Can you work these out from the model? Positions are in its coordinate system, mm. Face numbers are marked on the shaded views. A direction names the side the tool comes from. Give positions to 0.01 mm unless a question says otherwise; leave off trailing zeros. Order: outer loops, then holes, each group sorted by start corner. A loop starts at its lowest first (then second) coordinate and runs counter-clockwise, first axis right, second up. Notation, with made-up numbers: (84, 15.25) - (141, 15.25) arc R25 ccw to (141, 54.25) - close; hole circle Ø4 at (-5, 66.5). An arc over 180 degrees is marked (long way). Return JSON: item names as keys, results as strings.
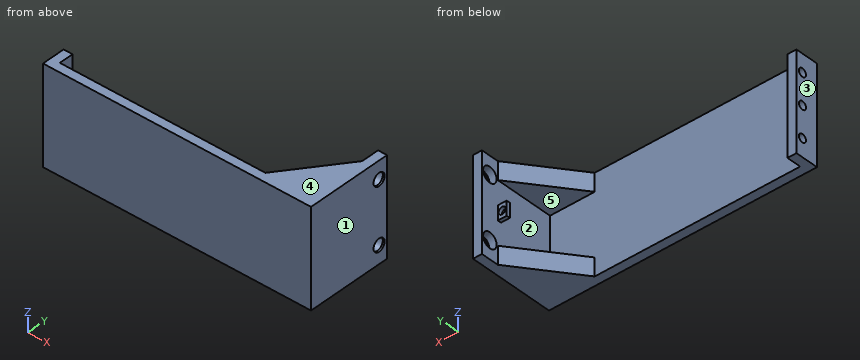
```python
from build123d import *

# Parameters (mm, degrees)
SKETCH1_W                 = 150
SKETCH1_H                 = 54.5
BOSS_EXTRUDE1_DEPTH       = 5
SKETCH2_W                 = 5
SKETCH2_H                 = 54.5
BOSS_EXTRUDE2_DEPTH       = 8
F_8_CLEARANCE_HOLE1_D     = 4.4958
F_8_CLEARANCE_HOLE1_DEPTH = 17
F_8_CLEARANCE_HOLE1_TIP   = 1.350674586
SKETCH7_W                 = 5
SKETCH7_H                 = 54.5
BOSS_EXTRUDE3_DEPTH       = 43
SKETCH8_R                 = 4.25
CUT_EXTRUDE1_DEPTH        = 4
RIB1_REACH                = 120.085
SKETCH10_WALL_W           = 279.571445908
SKETCH10_WALL_H           = 10
RIB3_REACH                = 120.085
SKETCH12_WALL_W           = 279.571445908
SKETCH12_WALL_H           = 10
SKETCH13_W                = 8
SKETCH13_H                = 2
BOSS_EXTRUDE4_DEPTH       = 5
SKETCH14_R                = 2
CUT_EXTRUDE2_DEPTH        = 2
SKETCH15_R                = 3.5
CUT_EXTRUDE3_DEPTH        = 1


with BuildPart() as part:
    # Sketch1 → Boss-Extrude1 (new body)
    with BuildSketch(Plane(origin=(0, 0, 0), x_dir=(1, 0, 0), z_dir=(0, 1, 0))):
        with Locations((-18.112463826, -1.689393939)):
            Rectangle(SKETCH1_W, SKETCH1_H)
    extrude(amount=BOSS_EXTRUDE1_DEPTH)

    # Sketch2 → Boss-Extrude2 (add)
    with BuildSketch(Plane(origin=(0, 5, 0), x_dir=(1, 0, 0), z_dir=(0, 1, 0))):
        with Locations((-90.612463826, -1.689393939)):
            Rectangle(SKETCH2_W, SKETCH2_H)
    extrude(amount=BOSS_EXTRUDE2_DEPTH)

    # #8 Clearance Hole1
    with Locations(Plane(origin=(-93.112463826, 9.2, -15.560606061), x_dir=(0, 0, -1), z_dir=(-1, 0, 0))):
        with Locations((0, 0), (-17.25, 0), (-34.5, 0)):
            Hole(F_8_CLEARANCE_HOLE1_D / 2, depth=F_8_CLEARANCE_HOLE1_DEPTH)
            with Locations((0, 0, -(F_8_CLEARANCE_HOLE1_DEPTH + F_8_CLEARANCE_HOLE1_TIP / 2))):  # 118° drill point
                Cone(0, F_8_CLEARANCE_HOLE1_D / 2, F_8_CLEARANCE_HOLE1_TIP, mode=Mode.SUBTRACT)

    # Sketch7 → Boss-Extrude3 (add)
    with BuildSketch(Plane(origin=(0, 5, 0), x_dir=(1, 0, 0), z_dir=(0, 1, 0))):
        with Locations((54.387536174, -1.689393939)):
            Rectangle(SKETCH7_W, SKETCH7_H)
    extrude(amount=BOSS_EXTRUDE3_DEPTH)

    # Sketch8 → Cut-Extrude1 (cut)
    with BuildSketch(Plane.ZY.offset(-51.887536174)):
        with Locations((-15.560606061, 43)):
            Circle(SKETCH8_R)
        with Locations((18.939393939, 43)):
            Circle(SKETCH8_R)
    extrude(amount=-CUT_EXTRUDE1_DEPTH, mode=Mode.SUBTRACT)

    # Sketch10 wall → Rib1 (add, up to next)
    with BuildSketch(Plane(origin=(39.387536174, 21.5, -25.560606061), x_dir=(-0.603857687995, -0.797092148154, 0), z_dir=(-0.797092148154, 0.603857687995, 0)), mode=Mode.PRIVATE) as rib1_sk1:
        with Locations((0, 5)):
            Rectangle(SKETCH10_WALL_W, SKETCH10_WALL_H)
    rib1_tool1 = extrude(rib1_sk1.sketch, amount=-RIB1_REACH, mode=Mode.PRIVATE) - part.part
    add(rib1_tool1.solids().sort_by_distance((39.387536174, 21.5, -25.560606061))[0])

    # Sketch12 wall → Rib3 (add, up to next)
    with BuildSketch(Plane(origin=(39.387536174, 21.5, 28.939393939), x_dir=(-0.603857687995, -0.797092148154, 0), z_dir=(0.797092148154, -0.603857687995, 0)), mode=Mode.PRIVATE) as rib3_sk1:
        with Locations((0, 5)):
            Rectangle(SKETCH12_WALL_W, SKETCH12_WALL_H)
    rib3_tool1 = extrude(rib3_sk1.sketch, amount=RIB3_REACH, mode=Mode.PRIVATE) - part.part
    add(rib3_tool1.solids().sort_by_distance((39.387536174, 21.5, 28.939393939))[0])

    # Sketch13 → Boss-Extrude4 (add)
    with BuildSketch(Plane.ZY.offset(-51.887536174)):
        with Locations((1.689393939, 37)):
            Rectangle(SKETCH13_W, SKETCH13_H)
    extrude(amount=BOSS_EXTRUDE4_DEPTH)

    # Sketch14 → Cut-Extrude2 (cut)
    with BuildSketch(Plane(origin=(0, 38, 0), x_dir=(1, 0, 0), z_dir=(0, 1, 0))):
        with Locations(Location((49.387536174, -1.689393939, 0), (0, 0, 270))):
            Circle(SKETCH14_R)
    extrude(amount=-CUT_EXTRUDE2_DEPTH, mode=Mode.SUBTRACT)

    # Sketch15 → Cut-Extrude3 (cut)
    with BuildSketch(Plane.ZY.offset(-55.887536174)):
        with Locations((-15.560606061, 43)):
            Circle(SKETCH15_R)
        with Locations((18.939393939, 43)):
            Circle(SKETCH15_R)
    extrude(amount=-CUT_EXTRUDE3_DEPTH, mode=Mode.SUBTRACT)


solid = part.part
```
1. Suppose I cut it at B-B (z = 11.5). List the corners of the cut face in (x, y) for me.
Checks:
{"outline": "(-93.11, 0) - (56.89, 0) - (56.89, 48) - (51.89, 48) - (51.89, 5) - (-88.11, 5) - (-88.11, 13) - (-93.11, 13) - close"}
2. Suppose I cut it at C-C (z = 1.5). List the corners of the cut face in (x, y) for me.
Checks:
{"outline": "(-93.11, 0) - (56.89, 0) - (56.89, 48) - (51.89, 48) - (51.89, 38) - (51.38, 38) - (51.38, 36) - (51.89, 36) - (51.89, 5) - (-88.11, 5) - (-88.11, 6.96) - (-93.11, 6.96) - close; (-93.11, 11.44) - (-88.11, 11.44) - (-88.11, 13) - (-93.11, 13) - close; (46.89, 36) - (47.4, 36) - (47.4, 38) - (46.89, 38) - close"}
3. Suppose I cut it at A-A (y = 43). List the corners of the cut face in (x, z) for me.
Checks:
{"outline": "(51.89, -25.56) - (56.89, -25.56) - (56.89, -19.06) - (55.89, -19.06) - (55.89, -19.81) - (51.89, -19.81) - close; (51.89, -11.31) - (55.89, -11.31) - (55.89, -12.06) - (56.89, -12.06) - (56.89, 15.44) - (55.89, 15.44) - (55.89, 14.69) - (51.89, 14.69) - close; (51.89, 23.19) - (55.89, 23.19) - (55.89, 22.44) - (56.89, 22.44) - (56.89, 28.94) - (51.89, 28.94) - close"}
4. If I drill on L1, parallel to Z at x = -91, y = 9.2; L2, parallel to Z at x = 51, y = 22; L3, parallel to Y at x = 17.5, z = -6, over which ranges is the centre line in solid material (lowest first)? Write a range as [from, to].
Checks:
{"L1": "[-25.56, -17.81], [-13.31, -0.56], [3.94, 16.69], [21.19, 28.94]", "L2": "[-25.56, -15.56], [18.94, 28.94]", "L3": "[0, 5]"}
5. Suppose I cut it at D-D (y = 9.2). List the corners of the cut face in (x, z) for me.
Checks:
{"outline": "(-93.11, -25.56) - (-88.11, -25.56) - (-88.11, -17.81) - (-93.11, -17.81) - close; (-93.11, -13.31) - (-88.11, -13.31) - (-88.11, -0.56) - (-93.11, -0.56) - close; (-93.11, 3.94) - (-88.11, 3.94) - (-88.11, 16.69) - (-93.11, 16.69) - close; (-93.11, 21.19) - (-88.11, 21.19) - (-88.11, 28.94) - (-93.11, 28.94) - close; (30.07, -25.56) - (56.89, -25.56) - (56.89, 28.94) - (30.07, 28.94) - (30.07, 18.94) - (51.89, 18.94) - (51.89, -15.56) - (30.07, -15.56) - close"}
6. On a 3-axis mill with a long thin cutter (end or side, diameter ignored), from which of +Z, -Z, +X, -X, +Y, -Y can I reach the whole of each face in a straight line? I mean the marked faces 1 and 2. Say none if no direction works.
Checks:
{"face 1": "+Z, -Z, +X, +Y, -Y", "face 2": "none"}
7. Thinking about a two-plate mould opening in X: for the marked faces 3, 4 and 5, which applies, +X half, -X half, draft (parallel to the pull), parting line (faces both ways), or undercut?
Checks:
{"face 3": "-X half", "face 4": "draft", "face 5": "undercut"}
8. For pin 1 Ø8 at (y, z) = (43, -15.56) entering from -X; pin 2 Ø1.6 at (x, y) = (48.5, 37) entering from -Z; pin 3 Ø12 at (x, z) = (-17, 2) entering from +Y, each with a flat end and sliding along its axis, tell me the tip position at first contact or that it passes through.
Checks:
{"pin 1": "x = 55.89", "pin 2": "z = -2.31", "pin 3": "y = 5"}
